Answer from the drawing. Dimensions are ordinates in mm from the lowest x, y and z of the part. A direction names the side the tool comes from. Round coordinates to 2 decimals unless told otherwise and drop trailing zeros. Write each loop counter-clockwise with the first axis right and the second up, starting at its lowest first coordinate (ties: lowest second). Pieces come first, ordered by that corner, then holes.
1. Find section B-B (y = 9.25). Write down the section's boundary in (x, z).
2. Flat-ended cylindrical pins translate along their axes: pin 1 Ø3.5 at (x, z) = (22.5, 9) entering from +Y; pin 2 Ø5 at (x, y) = (13.5, 19.5) entering from -Z; pin 3 Ø2.5 at (x, y) = (21.7, 9.25) entering from +Z; pin 4 Ø9 at (y, z) = (13, 12) entering from +X. Find the tip coordinate at first contact, or state that the pin passes through.
3. Straight lines are drawn through the part: probe 1 along Y at (x, z) = (21.7, 3.1); probe 2 along Z at (x, y) = (36, 7). For each, find the intervals that lie inside material, in ascending order.
4. Find section D-D (y = 27). Write down the section's boundary in (x, z), and give its area (3 significant figures).
5. Find section C-C (z = 9). Write down the section's boundary in (x, y).
6. Find section A-A (x = 21.7). Write down the section's boundary in (y, z).
7. A tool of negligible diameter and unlimited length cuts with its end or side. For the marked faces 1 and 2, from which of +Z, -Z, +X, -X, +Y, -Y can it reach the whole face along a straight path? Write none if from no direction.
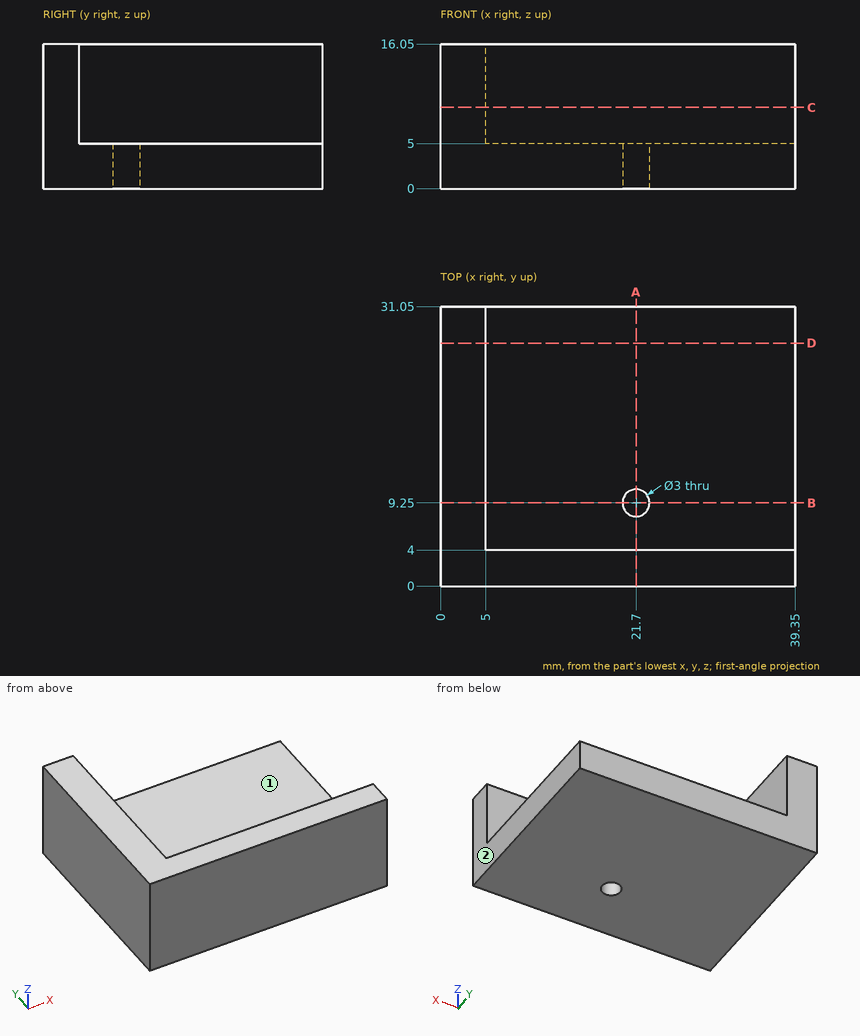
Worked answers:
1. outline: (0, 0) - (20.2, 0) - (20.2, 5) - (5, 5) - (5, 16.05) - (0, 16.05) - close; (23.2, 0) - (39.35, 0) - (39.35, 5) - (23.2, 5) - close
2. pin 1: stops at y = 4
2. pin 2: stops at z = 0
2. pin 3: passes through
2. pin 4: stops at x = 5
3. probe 1: y = 0 to 7.75, 10.75 to 31.05
3. probe 2: z = 0 to 5
4. outline: (0, 0) - (39.35, 0) - (39.35, 5) - (5, 5) - (5, 16.05) - (0, 16.05) - close
4. area: 252 mm2
5. outline: (0, 0) - (39.35, 0) - (39.35, 4) - (5, 4) - (5, 31.05) - (0, 31.05) - close
6. outline: (0, 0) - (7.75, 0) - (7.75, 5) - (4, 5) - (4, 16.05) - (0, 16.05) - close; (10.75, 0) - (31.05, 0) - (31.05, 5) - (10.75, 5) - close
7. face 1: +Z, +X, +Y
7. face 2: +Z, -Z, +X, +Y, -Y
